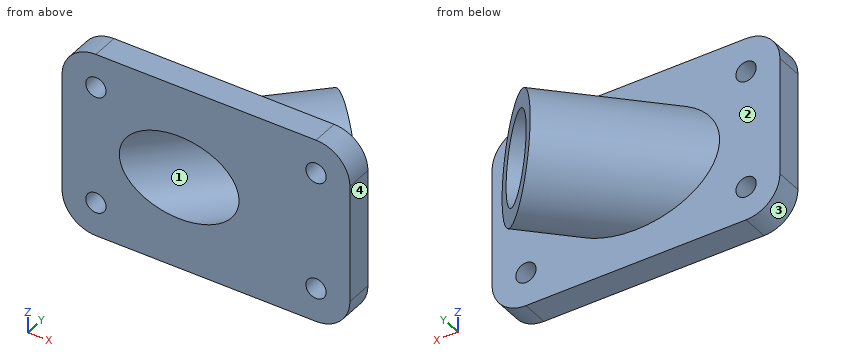
```python
from build123d import *

# Parameters (mm, degrees)
SKETCH1_W            = 107.95
SKETCH1_H            = 69.85
BOSS_EXTRUDE1_DEPTH  = 10.16
SKETCH3_R            = 3.81
CUT_EXTRUDE1_DEPTH   = 66.086725605
LPATTERN1_COUNT      = 20
LPATTERN1_PITCH      = 82.55
LPATTERN1_COUNT_DIR2 = 2
LPATTERN1_PITCH_DIR2 = 44.45
FILLET1_R            = 12.7
BOSS_EXTRUDE2_REACH  = 100.241
SKETCH4_R            = 22.225
SKETCH5_R            = 15.875
CUT_EXTRUDE2_DEPTH   = 99.241498296


with BuildPart() as part:
    # Sketch1 → Boss-Extrude1 (new body)
    with BuildSketch(Plane(origin=(0, 0, 0), x_dir=(1, 0, 0), z_dir=(0, 1, 0))):
        Rectangle(SKETCH1_W, SKETCH1_H)
    extrude(amount=BOSS_EXTRUDE1_DEPTH)

    # Sketch3 → Cut-Extrude1 (cut, through all)
    with BuildSketch(Plane(origin=(0, 10.16, 0), x_dir=(1, 0, 0), z_dir=(0, 1, 0))):
        with Locations(Location((41.275, 22.225, 0), (0, 0, 270))):
            Circle(SKETCH3_R)
    cut_extrude1 = extrude(amount=-CUT_EXTRUDE1_DEPTH, mode=Mode.SUBTRACT)

    # LPattern1: Cut-Extrude1 20 × 2
    with Locations(*[(-i * LPATTERN1_PITCH, 0, j * LPATTERN1_PITCH_DIR2) for i in range(LPATTERN1_COUNT) for j in range(LPATTERN1_COUNT_DIR2) if (i, j) != (0, 0)]):
        add(cut_extrude1, mode=Mode.SUBTRACT)

    # Fillet1
    fillet1_edges = [part.edges().sort_by_distance(p)[0] for p in [
        (53.975, 5.08, 34.925),
        (-53.975, 5.08, 34.925),
        (-53.975, 5.08, -34.925),
        (53.975, 5.08, -34.925),
    ]]
    fillet(fillet1_edges, radius=FILLET1_R)

    # Boss-Extrude2: up to this plane
    boss_extrude2_end = Plane(origin=(0, 10.16, 0), z_dir=(0, -1, 0))
    # Sketch4 → Boss-Extrude2 (add, up to the surface)
    with BuildSketch(Plane(origin=(32.0675, 32.0675, 0), x_dir=(0, 0, -1), z_dir=(0.7071067811865488, 0.7071067811865464, 0)), mode=Mode.PRIVATE) as boss_extrude2_sk1:
        with Locations(Location((0, 7.118116382, 0), (0, 0, 90))):
            Circle(SKETCH4_R)
    boss_extrude2_tool1 = split(extrude(boss_extrude2_sk1.sketch, amount=-BOSS_EXTRUDE2_REACH, mode=Mode.PRIVATE), bisect_by=boss_extrude2_end, keep=Keep.BOTH, mode=Mode.PRIVATE)
    add(boss_extrude2_tool1.solids().sort_by_distance((27.034232, 37.100768, 0))[0])

    # Sketch5 → Cut-Extrude2 (cut, through all)
    with BuildSketch(Plane(origin=(32.0675, 32.0675, 0), x_dir=(0, 0, -1), z_dir=(0.7071067811865488, 0.7071067811865464, 0))):
        with Locations(Location((0, 7.118116382, 0), (0, 0, 90))):
            Circle(SKETCH5_R)
    extrude(amount=-CUT_EXTRUDE2_DEPTH, mode=Mode.SUBTRACT)


solid = part.part
```
Verification items for the finished model (mm, model axes). Face numbers are marked on the shaded views. Round coordinates to 2 decimals unless told otherwise and drop trailing zeros. Order: outer loops, then holes, each group sorted by start corner. A loop starts at its lowest first (then second) coordinate and runs counter-clockwise, first axis right, second up. Notation, with made-up numbers: (10.5, 16.25) -> (22.5, 16.25) arc R19 cw to (22.5, 43.25) -> close; hole circle Ø2 at (2.25, 56.5). An arc over 180 degrees is marked (long way). Put each result on its own line as item: value. Start each with the question number.
(1) Section check B-B (y = 6.5). State how many separate pieces and enclosed holes the cut face has, then the cut area to 3 significant figures.
(2) Depth check by flat-ended pin: pin 1 Ø4 at (x, y) = (21.5, 11.5) entering from -Z (3 decimals); pin 2 Ø2 at (y, z) = (37.5, -4) entering from -X; pin 3 Ø4 at (y, z) = (27.5, 26) entering from -X; pin 4 Ø4 at (y, z) = (33, 21.5) entering from +X. Enter the tip coordinate at first touch or a pass-through.
(3) Draft check along X on the marked faces 1, 2, 3 and 4. Enter one of: +X half, -X half, draft (parallel to the pull), parting line (faces both ways), or undercut.
(4) Section check A-A (z = 3). Enter the section's corners in (x, y) (3 decimals), then the cut area to 3 significant figures.
(5) Material ranges on line 1 along Z through (x, y) = (-40, 4.5) (3 decimals); line 2 along Z through (x, y) = (12, 25); line 3 along Z through (x, y) = (14.5, 33.5), recorded low to high.
Completed:
1. separate pieces: 1
1. enclosed holes: 5
1. area: 6,100 mm2
2. pin 1: stops at z = -34.925
2. pin 2: stops at x = -4.52
2. pin 3: passes through
2. pin 4: stops at x = 32.92
3. face 1: undercut
3. face 2: draft
3. face 3: -X half
3. face 4: +X half
4. outline: (-53.975, 0) -> (-32.113, 0) -> (16.011, 48.124) -> (11.463, 52.672) -> (-31.05, 10.16) -> (-53.975, 10.16) -> close; (11.98, 0) -> (53.975, 0) -> (53.975, 10.16) -> (31.237, 10.16) -> (42.606, 21.529) -> (38.057, 26.078) -> close
4. area: 1,140 mm2
5. line 1: z = -34.925 to -25.815, -18.635 to 18.635, 25.815 to 34.925
5. line 2: z = -22.13 to -15.74, 15.74 to 22.13
5. line 3: z = -21.31 to -14.56, 14.56 to 21.31
